Autodesk Inventor part; units mm, degrees
ref_plane "YZ Plane" through (0, 0, 0) normal (1, 0, 0) x (0, 1, 0)
ref_plane "XZ Plane" through (0, 0, 0) normal (0, 1, 0) x (-1, 0, 0)
ref_plane "XY Plane" through (0, 0, 0) normal (0, 0, 1) x (1, 0, 0)
sketch "草圖1" plane through (0, 0, 0) normal (0, 1, 0) x (-1, 0, 0)
  line L0 (0, 0) -> (5, 0)
  line L1 (5, 0) -> (5, -20)
  line L2 (5, -20) -> (0, -20)
  line L3 (0, -20) -> (0, 0)
  dimension "d0" = 5
  dimension "d1" = 20
extrude "擠出1" add sketch "草圖1" along normal blind 20
sketch "草圖3" plane through (0, 20, 0) normal (0, 1, 0) x (1, 0, 0)
  line L0 (0, 20) -> (-5, 20)
  line L1 (0, 0) -> (-5, 0)
  line L2 (-5, 0) -> (-5, 20)
  line L3 (-5, 20) -> (0, 20)
  line L4 (0, 20) -> (0, 0)
extrude "擠出3" add sketch "草圖3" along normal blind 5
sketch "草圖4" plane through (-5, 0, 0) normal (0, 0, 1) x (1, 0, 0)
  line L0 (5, 0) -> (5, 25)
  line L1 (0, 25) -> (5, 25)
  line L2 (5, 25) -> (0, 25)
  line L3 (5, 25) -> (25, 32.5)
  line L4 (5, 20) -> (25, 12.5)
  line L5 (25, 12.5) -> (25, 32.5)
  line L6 (0, 0) -> (5, 0)
  line L7 (0, 0) -> (0, 25)
  line L8 (-5.1212, 0) -> (30.7273, 0)
  dimension "d8" = 5
  dimension "d9" = 20
  dimension "d19" = 20
extrude "擠出4" add sketch "草圖4" against normal up to surface (20 mm away) contours L0 L3 L5 L4
shell "薄殼2" thickness 1 removed faces 2 at (20, 19.1667, -6.6667) at (-1.6667, 0, -6.6667)
equation "\"d0\" = bottom_w"
equation "\"d1\" = bottom_l"
equation "\"d2\" = bottom_h"
equation "\"d6\" = nuzzle_lh"
equation "\"d8\" = nuzzle_lh"
equation "\"d9\" = 4 * nuzzle_lh"
equation "\"d15\" = nuzzle_lh"
equation "\"bottom_w\" = 5"
equation "\"bottom_l\" = 20"
equation "\"bottom_h\" = 20"
equation "\"nuzzle_lh\" = 5"
properties part number "nuzzle_v1_0310"
The model under review builds one solid part; all positions refer to its coordinate system, in mm. A direction names the side the tool comes from. Coordinates: 2 decimals unless noted, no trailing zeros. Loops run counter-clockwise (first coordinate to the right, second up) from the corner with the lowest first, then second, coordinate; pieces in that order, holes last. Notation, with made-up numbers: (69, -32) -> (117, -32) arc R25 cw to (117, -3) -> close; hole circle Ø10 at (-23, 64.25). An arc over 180 degrees is marked (long way). Use a Markdown table: item, result. Add a question column.
1. Add section D-D on y = 6.5. Write out the cut boundary in (x, z).
2. Add section C-C on x = 18.25. Write out the cut boundary in (y, z).
3. Add section A-A on z = -17. Write out the cut boundary in (x, y), plus the area to 3 significant figures.
4. Machinability: for faces 4 (the face through (9.952, 27.664, -9.874)), 5 (the face through (9, 20, -1)), 6 (the face through (-4, 12, -10)), which of the approach directions +Z, -Z, +X, -X, +Y, -Y give a long, thin tool a straight path to every point of the face, cutting with its end or side? Answer none if there is none.
5. Add section B-B on y = 21. Write out the cut boundary in (x, z), plus the area to 3 significant figures.
6. Clearance check with flat-ended pins moving along their axes: pin 1 Ø5.5 at (x, z) = (-1.5, -12) entering from +Y; pin 2 Ø1 at (x, z) = (0.5, -2.5) entering from +Y (3 decimals); pin 3 Ø5 at (x, z) = (4.5, -6) entering from -Y (3 decimals). State where each tip first meets the part, or that it passes through.
7. Draft analysis for pull direction Y (two halves, no side actions). For faces 1 (the face through (9.86, 16.302, -9.86)), 2 (the face through (-2, 24, -10)), 3 (the face through (-1, 11, -10)), state which applies: pulls with the +Y half, pulls with the -Y half, needs draft (parallel to the pull), parting line crosses it, or undercut.
8. To check wall thickness, follow line 1 (Z direction, x = 8, y = 21); line 2 (X direction, y = 10, z = -13.25); line 3 (Y direction, x = 2, z = -2.5). State the ranges of each line that lie inside material, in increasing order.
Returned:
| question | item | result |
|---|---|---|
| 1 | outline | (-5, -20) -> (0, -20) -> (0, 0) -> (-5, 0) -> close; hole (-4, -19) -> (-1, -19) -> (-1, -1) -> (-4, -1) -> close |
| 2 | outline | (13.16, -20) -> (31.84, -20) -> (31.84, 0) -> (13.16, 0) -> close; hole (14.22, -19) -> (30.78, -19) -> (30.78, -1) -> (14.22, -1) -> close |
| 3 | outline | (-5, 0) -> (-4, 0) -> (-4, 24) -> (0.18, 24) -> (20, 31.43) -> (20, 32.5) -> (0, 25) -> (-5, 25) -> close; (-1, 0) -> (0, 0) -> (0, 20) -> (20, 12.5) -> (20, 13.57) -> (-1, 21.44) -> close |
| 3 | area | 93.0 mm² |
| 4 | face 4 | +X |
| 4 | face 5 | none |
| 4 | face 6 | -Y |
| 5 | outline | (-5, -20) -> (20, -20) -> (20, -19) -> (0.18, -19) -> (0.18, -1) -> (20, -1) -> (20, 0) -> (-5, 0) -> close; hole (-4, -19) -> (-1, -19) -> (-1, -1) -> (-4, -1) -> close |
| 5 | area | 89.3 mm² |
| 6 | pin 1 | stops at y = 25.47 |
| 6 | pin 2 | stops at y = 25.375 |
| 6 | pin 3 | stops at y = 17.375 |
| 7 | face 1 | pulls with the -Y half |
| 7 | face 2 | undercut |
| 7 | face 3 | needs draft |
| 8 | line 1 | z = -20 to -19, -1 to 0 |
| 8 | line 2 | x = -5 to -4, -1 to 0 |
| 8 | line 3 | y = 19.25 to 20.32, 24.68 to 25.75 |
